Check sheet for the modelled part. Datum: model origin and axes. Units: mm. A direction names the side the tool comes from. Round coordinates to 2 decimals unless told otherwise and drop trailing zeros. Write each loop counter-clockwise with the first axis right and the second up, starting at its lowest first coordinate (ties: lowest second). Pieces come first, ordered by that corner, then holes. Notation, with made-up numbers: (20, 21) -> (47, 21) arc R15 ccw to (47, 45) -> close; hole circle Ø9 at (-10, 81.5). An arc over 180 degrees is marked (long way). One line per item, written item: value.
Autodesk Inventor part; units mm, degrees
ref_plane "YZ Plane" through (0, 0, 0) normal (1, 0, 0) x (0, 1, 0)
ref_plane "XZ Plane" through (0, 0, 0) normal (0, 1, 0) x (-1, 0, 0)
ref_plane "XY Plane" through (0, 0, 0) normal (0, 0, 1) x (1, 0, 0)
sketch "Sketch1" plane through (0, 0, 0) normal (0, 1, 0) x (-1, 0, 0)
  circle A0 centre (0, 0) radius 14.224
  dimension "d0" = 28.448
extrude "Extrusion1" add sketch "Sketch1" along normal blind 6.35
sketch "Sketch2" plane through (0, 6.35, 0) normal (0, 1, 0) x (1, 0, 0)
  circle A0 centre (0, 0) radius 14.224
  circle A1 centre (0, 0) radius 11.8999
  dimension "d3" = 23.7998
extrude "Extrusion2" add sketch "Sketch2" along normal blind 12.7 contours A1
sketch "Sketch3" plane through (0, 19.05, 0) normal (0, 1, 0) x (1, 0, 0)
  circle A0 centre (0, 0) radius 11.8999
  circle A1 centre (0, 0) radius 6.35
  dimension "d6" = 12.7
extrude "Extrusion3" cut sketch "Sketch3" against normal blind 2540 contours A1
thread "Thread1"
thread "Thread2"
properties part number "ACME Threaded Rod Nut" material "Bronze, Cast"
Item 1: Depth check by flat-ended pin: P1, Ø2, axis at y = 15.5, z = -2, coming from the -X side; P2, Ø6, axis at y = 14, z = 7, coming from the +X side; P3, Ø3, axis at y = 7.5, z = 5, coming from the +X side. Enter the tip coordinate at first touch or a pass-through.
Answer:
P1: stops at x = -11.86
P2: stops at x = 11.21
P3: stops at x = 13.64
Item 2: Mould release check, pull along Z, two halves, no side actions. Record for faces 1 (the flat face through (-6, 0, -3)), 2 (the cylindrical face through (-1.38, 9.66, 6.2)), 3 (the cylindrical face through (-9.443, 12.611, -7.241)): pulls with the +Z half, pulls with the -Z half, needs draft (parallel to the pull), parting line crosses it, or undercut.
Answer:
face 1: needs draft
face 2: undercut
face 3: parting line crosses it
Item 3: Sectioned sample at D-D on x = 9.5. Enter the section's corners in (y, z), and give its area (3 significant figures).
Answer:
outline: (0, -10.59) -> (6.35, -10.59) -> (6.35, -7.17) -> (19.05, -7.17) -> (19.05, 7.17) -> (6.35, 7.17) -> (6.35, 10.59) -> (0, 10.59) -> close
area: 316 mm^2
Item 4: Sectioned sample at A-A on x = 0. Enter the section's corners in (y, z).
Answer:
outline: (0, -14.22) -> (6.35, -14.22) -> (6.35, -11.9) -> (19.05, -11.9) -> (19.05, -6.35) -> (0, -6.35) -> close; (0, 6.35) -> (19.05, 6.35) -> (19.05, 11.9) -> (6.35, 11.9) -> (6.35, 14.22) -> (0, 14.22) -> close
Item 5: Tool access check on faces 4 (the flat face through (5, 19.05, 5)), 5 (the flat face through (3, 6.35, -12)). Record the directions out of +Z, -Z, +X, -X, +Y, -Y that give a thin tool (end or side, any length) a straight path to the whole face; none if there is none.
Answer:
face 4: +Z, -Z, +X, -X, +Y
face 5: +Y
Item 6: Thickness scan on line 1 (Z direction, x = 0, y = 5); line 2 (X direction, y = 11, z = 0). Record the ranges inside material, lowest first.
Answer:
line 1: z = -14.22 to -6.35, 6.35 to 14.22
line 2: x = -11.9 to -6.35, 6.35 to 11.9
Item 7: Sectioned sample at C-C on y = 2.25. Enter the section's corners in (x, z).
Answer:
outline: circle Ø28.45 at (0, 0); hole circle Ø12.7 at (0, 0)
Item 8: Sectioned sample at B-B on z = 0. Enter the section's corners in (x, y), and give its area (3 significant figures).
Answer:
outline: (-14.22, 0) -> (-6.35, 0) -> (-6.35, 19.05) -> (-11.9, 19.05) -> (-11.9, 6.35) -> (-14.22, 6.35) -> close; (6.35, 0) -> (14.22, 0) -> (14.22, 6.35) -> (11.9, 6.35) -> (11.9, 19.05) -> (6.35, 19.05) -> close
area: 241 mm^2
